Geometry: final body of the model. Coordinates: model frame, mm. Face numbers are marked on the shaded views. Round coordinates to 2 decimals unless told otherwise and drop trailing zeros. Write each loop counter-clockwise with the first axis right and the second up, starting at its lowest first coordinate (ties: lowest second). Pieces come first, ordered by that corner, then holes. Notation, with made-up numbers: (10, 15.5) -> (49, 15.5) arc R20 ccw to (49, 29.5) -> close; hole circle Ø8 at (37, 18.25). An arc over 180 degrees is marked (long way). One line per item, written item: value. Start each with the question number.
from build123d import *

# Parameters (mm, degrees)
F0_R            = 40
F1_DEPTH        = 8
F2_R            = 9.5
F3_DEPTH        = 8.001
F6_R            = 2
F7_DEPTH        = 15
F7_COPIES_COUNT = 4


# Not quite as in the source:
# - a pattern or mirror of a feature is missing from the dataset's text; its kind, count and spacing are read off the source's solid


with BuildPart() as f1:
    # F0 (on Top) → F1 (new body)
    with BuildSketch(Plane.XY):
        Circle(F0_R)
    extrude(amount=F1_DEPTH)

    # F2 (on face) → F3 (cut, through all)
    with BuildSketch(Plane.XY.offset(8)):
        Circle(F2_R)
    extrude(amount=-F3_DEPTH, mode=Mode.SUBTRACT)

    # F6 (on offset) → F7 (cut)
    with BuildSketch(Plane.XZ.offset(40.792)):
        with Locations((0, 4)):
            Circle(F6_R)
    f7 = extrude(amount=-F7_DEPTH, mode=Mode.SUBTRACT)

    # F7_copies: F7 ×4 about axis
    f7_copies_axis = Axis((0, 0, 0), (0, 0, 1))
    for i in range(1, F7_COPIES_COUNT):
        add(f7.rotate(f7_copies_axis, i * 360 / F7_COPIES_COUNT), mode=Mode.SUBTRACT)


solid = f1.part
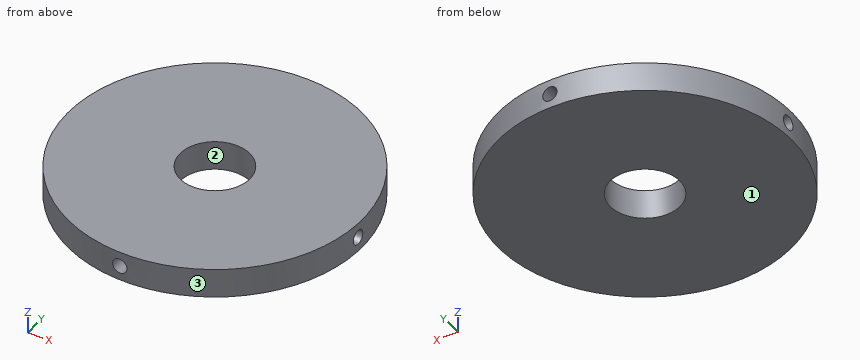
(1) Line query: probe 1 along Z at (x, y) = (0, -33); probe 2 along X at (y, z) = (4, 4); probe 3 along Y at (x, z) = (-0.5, 4.5). Output: solid intervals per line, ascending.
(2) Section query A-A (x = 0). Output: boundary loops of the cut face in (y, z).
(3) Pull-direction query (Y, two-part tool) for the marked faces 1, 2 and 3; classes: pulls with the +Y half, pulls with the -Y half, needs draft (parallel to the pull), parting line crosses it, or undercut.
(4) Section query D-D (y = -18.5). Output: boundary loops of the cut face in (x, z).
(5) Section query C-C (y = -33.5). Output: boundary loops of the cut face in (x, z), and give its area (3 significant figures).
(6) Pin query (flat end, axial travel): pin 1 (2 mm diameter, centred on y = 0.5, z = 4.5, fed in from -X); pin 2 (2.5 mm diameter, centred on x = 0, z = 4, fed in from -Y); pin 3 (2 mm diameter, centred on x = 0, z = 3.5, fed in from +Y). Return the tip coordinate at first contact, or that it passes through.
Results list:
1. probe 1: z = 0 to 2, 6 to 8
1. probe 2: x = -39.8 to -8.62, 8.62 to 39.8
1. probe 3: y = -25.79 to -9.49, 9.49 to 25.79
2. outline: (-40, 0) -> (-9.5, 0) -> (-9.5, 8) -> (-40, 8) -> (-40, 6) -> (-25.79, 6) -> (-25.79, 2) -> (-40, 2) -> close; (9.5, 0) -> (40, 0) -> (40, 2) -> (25.79, 2) -> (25.79, 6) -> (40, 6) -> (40, 8) -> (9.5, 8) -> close
3. face 1: needs draft
3. face 2: undercut
3. face 3: parting line crosses it
4. outline: (-35.46, 0) -> (35.46, 0) -> (35.46, 8) -> (-35.46, 8) -> close
5. outline: (-21.86, 0) -> (21.86, 0) -> (21.86, 8) -> (-21.86, 8) -> close; hole circle Ø4 at (0, 4)
5. area: 337 mm^2
6. pin 1: stops at x = -25.79
6. pin 2: stops at y = -25.79
6. pin 3: stops at y = 25.79
